```python
from build123d import *

# Parameters (mm, degrees)
F2_R     = 75
F2_W     = 50
F2_H     = 50
F3_DEPTH = 2


# Not quite as in the source:
# - a feature of the source that left no trace in its solid (it failed there, or was rolled back) is left out


with BuildPart() as f3:
    # F2 (on offset) → F3 (new body)
    with BuildSketch(Plane.XZ.offset(60)):
        Circle(F2_R)
        Polygon((-45, 15), (-45, 0), (-45, -15), (-51, -15), (-51, 15), align=None, mode=Mode.SUBTRACT)
        Rectangle(F2_W, F2_H, mode=Mode.SUBTRACT)
        Polygon((45, -15), (45, 0), (45, 15), (51, 15), (51, -15), align=None, mode=Mode.SUBTRACT)
    extrude(amount=F3_DEPTH)


solid = f3.part
```
Can you work these out from the model? Positions are in its coordinate system, mm. Coordinates: 2 decimals unless noted, no trailing zeros. Loops run counter-clockwise (first coordinate to the right, second up) from the corner with the lowest first, then second, coordinate; pieces in that order, holes last.
Item 1: Suppose I cut it at B-B (y = -61.2). Please give me the cut outline in (x, z).
Answers below:
outline: circle Ø150 at (0, 0); hole (-51, -15) - (-45, -15) - (-45, 15) - (-51, 15) - close; hole (-25, -25) - (25, -25) - (25, 25) - (-25, 25) - close; hole (45, -15) - (51, -15) - (51, 15) - (45, 15) - close
Item 2: Suppose I cut it at D-D (x = 16). Please give me the cut outline in (y, z).
Answers below:
outline: (-62, -73.27) - (-60, -73.27) - (-60, -25) - (-62, -25) - close; (-62, 25) - (-60, 25) - (-60, 73.27) - (-62, 73.27) - close
Item 3: Suppose I cut it at A-A (z = 0). Please give me the cut outline in (x, y).
Answers below:
outline: (-75, -62) - (-51, -62) - (-51, -60) - (-75, -60) - close; (-45, -62) - (-25, -62) - (-25, -60) - (-45, -60) - close; (25, -62) - (45, -62) - (45, -60) - (25, -60) - close; (51, -62) - (75, -62) - (75, -60) - (51, -60) - close
Item 4: Please list where these lines run through material, in increasing order: L1, parallel to X at y = -60.2, z = -0.5; L2, parallel to X at y = -61.75, z = -7; L3, parallel to X at y = -61, z = 24.
Answers below:
L1: x = -75 to -51, -45 to -25, 25 to 45, 51 to 75
L2: x = -74.67 to -51, -45 to -25, 25 to 45, 51 to 74.67
L3: x = -71.06 to -25, 25 to 71.06
Item 5: Suppose I cut it at C-C (x = 0). Please give me the cut outline in (y, z).
Answers below:
outline: (-62, -75) - (-60, -75) - (-60, -25) - (-62, -25) - close; (-62, 25) - (-60, 25) - (-60, 75) - (-62, 75) - close
Item 6: I'm going to push flat-ended pins straight in: pin 1 (0.6 mm diameter, centred on x = 7.5, y = -61, fed in from -Z); pin 2 (0.6 mm diameter, centred on x = 47, y = -60.5, fed in from -Z); pin 3 (1 mm diameter, centred on x = 14.5, y = -61, fed in from -Z). Where does each tip first touch, or does it pass through?
Answers below:
pin 1: stops at z = -74.65
pin 2: stops at z = -58.69
pin 3: stops at z = -73.68
